Geometry check sheet. Reference: the model listing, model coordinates, mm. A direction names the side the tool comes from. Round coordinates to 2 decimals unless told otherwise and drop trailing zeros. Write each loop counter-clockwise with the first axis right and the second up, starting at its lowest first coordinate (ties: lowest second). Pieces come first, ordered by that corner, then holes. Notation, with made-up numbers: (34, -6.75) -> (87, -6.75) arc R16 ccw to (87, 7.25) -> close; hole circle Ø9 at (14, 48.25). An arc over 180 degrees is marked (long way). Return JSON: item names as keys, results as strings. Group by question number.
from build123d import *

# Parameters (mm, degrees)
PATTERN_CIRCULAR_1_COUNT = 2
PATTERN_CIRCULAR_1_ANGLE = 90
CHAMFER_1_SIZE           = 0.5
MOVE_BODY_1_ANGLE        = 90


with BuildPart() as part:
    # Эскиз1 → Повернуть1 (revolve)
    with BuildSketch(Plane.XY, mode=Mode.PRIVATE) as revolve_1_sk:
        Polygon((0, 2.8), (0.35, 2.8), (1.65, 1.5), (20, 1.5), (20, 0), (0, 0), align=None)
    revolve(revolve_1_sk.sketch.rotate(Axis((-6.35, 0, 0), (1, 0, 0)), 90), axis=Axis((-6.35, 0, 0), (1, 0, 0)))

    # Эскиз2 → Вырез-По сечениям1 section 0
    with BuildSketch(Plane.ZY):
        with BuildLine():
            Line((-0.37, 1.5), (0.37, 1.5))
            Line((0.37, 1.5), (0.37, -1.5))
            Line((0.37, -1.5), (-0.37, -1.5))
            Line((-0.37, -1.5), (-0.37, 1.5))
        make_face()
    # Эскиз3 → Вырез-По сечениям1 section 1
    with BuildSketch(Plane.ZY.offset(-2.1)):
        with BuildLine():
            Line((-0.37, 0.498), (0.37, 0.498))
            Line((0.37, 0.498), (0.37, -0.498))
            Line((0.37, -0.498), (-0.37, -0.498))
            Line((-0.37, -0.498), (-0.37, 0.498))
        make_face()
    loft_1 = loft(mode=Mode.SUBTRACT)

    # Круговой массив1: Вырез-По сечениям1 ×2 about axis
    pattern_circular_1_axis = Axis((0, 0, 0), (-1, 0, 0))
    for i in range(1, PATTERN_CIRCULAR_1_COUNT):
        add(loft_1.rotate(pattern_circular_1_axis, i * PATTERN_CIRCULAR_1_ANGLE / (PATTERN_CIRCULAR_1_COUNT - 1)), mode=Mode.SUBTRACT)

    # Эскиз4 → Вырез-Повернуть1 (revolve, cut)
    with BuildSketch(Plane.XY, mode=Mode.PRIVATE) as cut_revolve_1_sk:
        Polygon((0, 0), (0, 0.556), (2.1, 0.409153695), (2.232942094, 0), align=None)
    revolve(cut_revolve_1_sk.sketch.rotate(Axis((-0.899228133, 0, 0), (-1, 0, 0)), 270), axis=Axis((-0.899228133, 0, 0), (-1, 0, 0)), mode=Mode.SUBTRACT)

    # Фаска1
    chamfer_1_edges = [part.edges().sort_by_distance(p)[0] for p in [
        (20, 0, -1.5),
    ]]
    chamfer(chamfer_1_edges, length=CHAMFER_1_SIZE)


with BuildPart() as part_1:
    # Move Body 1: moved
    add(part.part.rotate(Axis((0, 0, 0), (0, 1, 0)), MOVE_BODY_1_ANGLE))


solid = part_1.part
1) Material ranges on probe 1 along X at (y, z) = (-0.1, -15.5); probe 2 along Y at (x, z) = (1.25, -14.25); probe 3 along Y at (x, z) = (-1.3, -17), recorded low to high. Write a range as [from, to].
2) Tool access check on faces 4 (the face through (-2.8, -0.1, -0.2)), 5 (the face through (-0.005, 0.992, -1.065)). Record the directions out of +Z, -Z, +X, -X, +Y, -Y that give a thin tool (end or side, any length) a straight path to the whole face; none if there is none.
3) Go/stop test with a flat-tipped pin: P1, Ø3, axis at x = 1.5, z = -6.5, coming from the -Y side. Record where the tip stops, or that it passes through.
4) Mould release check, pull along Y, two halves, no side actions. Record for faces 1 (the face through (0.005, -0.992, -1.065)), 2 (the face through (1.43, -0.45, -10.7)), 3 (the face through (0, 0, -20)): +Y half, -Y half, draft (parallel to the pull), parting line (faces both ways), or undercut.
5) Sectioned sample at A-A on z = -10.75. Enter the section's corners in (x, y), and give its area (3 significant figures).
Evaluation:
{
 "1": {"probe 1": "x = [-1.5, 1.5]", "probe 2": "y = [-0.83, 0.83]", "probe 3": "y = [-0.75, 0.75]"},
 "2": {"face 4": "+Z, -Z", "face 5": "+Z"},
 "3": {"P1": "stops at y = -1.5"},
 "4": {"face 1": "undercut", "face 2": "parting line", "face 3": "draft"},
 "5": {"outline": "circle Ø3 at (0, 0)", "area": "7.07 mm2"}
}
